from build123d import *

# Parameters (mm, degrees)
ESQUISSE1_R                                      = 22
BOSS_EXTRU_1_DEPTH                               = 7
ENL_V_MAT_EXTRU_1_REACH                          = 33.89
R_P_TITION_CIRCULAIRE1_COUNT                     = 5
ENL_V_MAT_EXTRU_2_REACH                          = 33.89
ESQUISSE6_R                                      = 3.3
CHAMBRAGE_POUR_VIS_T_TE_RONDE_BOMB_E_D           = 3.6576
CHAMBRAGE_POUR_VIS_T_TE_RONDE_BOMB_E_CBORE_D     = 7.54126
CHAMBRAGE_POUR_VIS_T_TE_RONDE_BOMB_E_CBORE_DEPTH = 2.4638


with BuildPart() as part:
    # Esquisse1 → Boss.-Extru.1 (new body)
    with BuildSketch(Plane(origin=(0, 0, 0), x_dir=(0, 0, -1), z_dir=(1, 0, 0))):
        Circle(ESQUISSE1_R)
    extrude(amount=BOSS_EXTRU_1_DEPTH)

    # Esquisse5 → Enlèv. mat.-Extru.1 (cut, up to next)
    with BuildSketch(Plane(origin=(7, 0, 0), x_dir=(0, 0, -1), z_dir=(1, 0, 0)), mode=Mode.PRIVATE) as enl_v_mat_extru_1_sk1:
        with BuildLine():
            Line((2.1, -20), (2.1, -24))
            ThreePointArc((2.1, -24), (0, -26.1), (-2.1, -24))
            Line((-2.1, -24), (-2.1, -20))
            ThreePointArc((-2.1, -20), (0, -17.9), (2.1, -20))
        make_face()
    enl_v_mat_extru_1_tool1 = extrude(enl_v_mat_extru_1_sk1.sketch, amount=-ENL_V_MAT_EXTRU_1_REACH, mode=Mode.PRIVATE) & part.part
    enl_v_mat_extru_1 = enl_v_mat_extru_1_tool1.solids().sort_by_distance((7, -22, 0))[0]
    add(enl_v_mat_extru_1, mode=Mode.SUBTRACT)

    # Répétition circulaire1: Enlèv. mat.-Extru.1 ×5 about axis
    r_p_tition_circulaire1_axis = Axis((0, 0, 0), (1, 0, 0))
    for i in range(1, R_P_TITION_CIRCULAIRE1_COUNT):
        add(enl_v_mat_extru_1.rotate(r_p_tition_circulaire1_axis, i * 360 / R_P_TITION_CIRCULAIRE1_COUNT), mode=Mode.SUBTRACT)

    # Esquisse6 → Enlèv. mat.-Extru.2 (cut, up to next)
    with BuildSketch(Plane(origin=(7, 0, 0), x_dir=(0, 0, -1), z_dir=(1, 0, 0)), mode=Mode.PRIVATE) as enl_v_mat_extru_2_sk1:
        Circle(ESQUISSE6_R)
    enl_v_mat_extru_2_tool1 = extrude(enl_v_mat_extru_2_sk1.sketch, amount=-ENL_V_MAT_EXTRU_2_REACH, mode=Mode.PRIVATE) & part.part
    add(enl_v_mat_extru_2_tool1.solids().sort_by_distance((7, 0, 0))[0], mode=Mode.SUBTRACT)

    # Chambrage pour vis à tête ronde bombée #61 (through all)
    with Locations(Plane.ZY):
        with Locations((-6.914797213, 6.914797213), (6.914797213, 6.914797213), (6.914797213, -6.914797213), (-6.914797213, -6.914797213)):
            CounterBoreHole(CHAMBRAGE_POUR_VIS_T_TE_RONDE_BOMB_E_D / 2, CHAMBRAGE_POUR_VIS_T_TE_RONDE_BOMB_E_CBORE_D / 2, CHAMBRAGE_POUR_VIS_T_TE_RONDE_BOMB_E_CBORE_DEPTH)


solid = part.part
Read the model definition and answer for the solid it produces. Units are mm, in the model's axes. A direction names the side the tool comes from. Give positions to 0.01 mm unless a question says otherwise; leave off trailing zeros. Loops run counter-clockwise (first coordinate to the right, second up) from the corner with the lowest first, then second, coordinate; pieces in that order, holes last. Notation, with made-up numbers: (6, 75.25) -> (15, 75.25) arc R15 ccw to (15, 97.25) -> close; hole circle Ø1 at (-12, 35.5). An arc over 180 degrees is marked (long way). Use a Markdown table: item, result.
Q1. Each of these flat-tipped pins is pushed along its axis until it touches: pin 1 (3 mm diameter, centred on y = -10, z = 2.5, fed in from -X); pin 2 (5 mm diameter, centred on y = 6.91, z = 6.91, fed in from -X); pin 3 (1.5 mm diameter, centred on x = 2, y = -20.5, fed in from -Z); pin 4 (1.5 mm diameter, centred on y = 17, z = 11.5, fed in from -X). Where does it stop, or does it pass through?
Solved:
| item | result |
|---|---|
| pin 1 | stops at x = 0 |
| pin 2 | stops at x = 2.46 |
| pin 3 | stops at z = -9.69 |
| pin 4 | passes through |
Q2. Section D-D, the plane x = 6.25 is taken. Determine the outline of the cut face in (y, z), then the cut area to 3 significant figures.
Solved:
| item | result |
|---|---|
| outline | (-21.9, -2.1) arc R22 ccw to (-8.76, -20.18) -> (-8.18, -18.37) arc R2.1 cw to (-4.18, -19.67) -> (-4.77, -21.48) arc R22 ccw to (16.48, -14.57) -> (14.95, -13.45) arc R2.1 cw to (17.41, -10.06) -> (18.95, -11.17) arc R22 ccw to (18.95, 11.17) -> (17.41, 10.06) arc R2.1 cw to (14.95, 13.45) -> (16.48, 14.57) arc R22 ccw to (-4.77, 21.48) -> (-4.18, 19.67) arc R2.1 cw to (-8.18, 18.37) -> (-8.76, 20.18) arc R22 ccw to (-21.9, 2.1) -> (-20, 2.1) arc R2.1 cw to (-20, -2.1) -> close; hole circle Ø3.66 at (-6.91, -6.91); hole circle Ø3.66 at (-6.91, 6.91); hole circle Ø6.6 at (0, 0); hole circle Ø3.66 at (6.91, -6.91); hole circle Ø3.66 at (6.91, 6.91) |
| area | 1,370 mm^2 |
Q3. Section B-B, the plane y = 0 is taken. Determine the outline of the cut face in (x, z).
Solved:
| item | result |
|---|---|
| outline | (0, -22) -> (7, -22) -> (7, -3.3) -> (0, -3.3) -> close; (0, 3.3) -> (7, 3.3) -> (7, 22) -> (0, 22) -> close |
Q4. Find the intervals of material crossed by line 1 along Z through (x, y) = (5, 8); line 2 along Z through (x, y) = (1.5, 8.5); line 3 along Y through (x, z) = (5, 0), in increasing order.
Solved:
| item | result |
|---|---|
| line 1 | z = -20.49 to -8.39, -5.44 to 5.44, 8.39 to 20.49 |
| line 2 | z = -20.29 to -10.34, -3.49 to 3.49, 10.34 to 20.29 |
| line 3 | y = -17.9 to -3.3, 3.3 to 22 |
Q5. Section C-C, the plane z = -8 is taken. Determine the outline of the cut face in (x, y), then the cut area to 3 significant figures.
Solved:
| item | result |
|---|---|
| outline | (0, -20.49) -> (7, -20.49) -> (7, -8.39) -> (2.46, -8.39) -> (2.46, -10.53) -> (0, -10.53) -> close; (0, -3.3) -> (2.46, -3.3) -> (2.46, -5.44) -> (7, -5.44) -> (7, 5.44) -> (2.46, 5.44) -> (2.46, 3.3) -> (0, 3.3) -> close; (0, 10.53) -> (2.46, 10.53) -> (2.46, 8.39) -> (7, 8.39) -> (7, 20.49) -> (0, 20.49) -> close |
| area | 225 mm^2 |
Q6. Section A-A, the plane z = 0 is taken. Determine the outline of the cut face in (x, y).
Solved:
| item | result |
|---|---|
| outline | (0, -17.9) -> (7, -17.9) -> (7, -3.3) -> (0, -3.3) -> close; (0, 3.3) -> (7, 3.3) -> (7, 22) -> (0, 22) -> close |
Q7. A tool of negligible diameter and unlimited length cuts with its end or side. For faces 1 (the face through (4, -21, 2.1)), 2 (the face through (3.549, -4.473, -20.561)), 3 (the face through (2.464, -6, -5)), 4 (the face through (3.451, 6.954, 20.872)), from which of +Z, -Z, +X, -X, +Y, -Y can it reach the whole face along a straight path? Write none if from no direction.
Solved:
| item | result |
|---|---|
| face 1 | +X, -X, -Y |
| face 2 | +X, -X |
| face 3 | -X |
| face 4 | +Z, +X, -X |
Q8. Determine the mould class of faces 5 (the face through (3.549, 18.172, -10.607)), 6 (the face through (1.215, -10.596, -7.732)), 7 (the face through (3, 22, 0)), 8 (the face through (3.55, 18.19, 10.62)) for opening direction Z: pulls with the +Z half, pulls with the -Z half, needs draft (parallel to the pull), parting line crosses it, or undercut.
Solved:
| item | result |
|---|---|
| face 5 | pulls with the -Z half |
| face 6 | undercut |
| face 7 | parting line crosses it |
| face 8 | pulls with the +Z half |
